Autodesk Inventor part; units mm, degrees
ref_plane "YZ Plane" through (0, 0, 0) normal (1, 0, 0) x (0, 1, 0)
ref_plane "XZ Plane" through (0, 0, 0) normal (0, 1, 0) x (-1, 0, 0)
ref_plane "XY Plane" through (0, 0, 0) normal (0, 0, 1) x (1, 0, 0)
sketch "Sketch1" plane through (0, 0, 0) normal (1, 0, 0) x (0, 1, 0)
  line L0 (0, 0) -> (-20, 0)
  line L1 (-20, 0) -> (-20, -20)
  line L2 (-20, -20) -> (0, -20)
  line L3 (0, -20) -> (0, 0)
  line L4 (0, -20) -> (4, -20)
  line L5 (4, -20) -> (4, 0)
  line L6 (4, 0) -> (0, 0)
  line L7 (0, 0) -> (0, -20)
  line L8 (4, 0) -> (0, 0)
  line L9 (0, 0) -> (0, 4)
  line L10 (0, 4) -> (4, 4)
  line L11 (4, 4) -> (4, 0)
  line L12 (0, 4) -> (-20, 4)
  line L13 (-20, 4) -> (-20, 0)
  line L14 (-20, 0) -> (0, 0)
  line L15 (0, 0) -> (0, 4)
  dimension "d0" = 20
  dimension "d1" = 20
  dimension "d2" = 4
  dimension "d3" = 4
extrude "Extrusion1" add sketch "Sketch1" along normal blind 40 contours L6 L5 L4 L3 | L9 L10 L11 L6 | L0 L13 L12 L9
sketch "Sketch2" plane through (0, -20, 4) normal (0, 0, 1) x (1, 0, 0)
  line L0 (0, 0) -> (40, 0)
  line L1 (20, 0) -> (20, 10)
  circle A0 centre (20, 10) radius 3.25
  point P0 (0, 20)
  dimension "d6" = 10
  dimension "d7" = 6.5
extrude "Extrusion2" cut sketch "Sketch2" against normal through all
sketch "Sketch3" plane through (0, -20, 4) normal (0, 0, 1) x (1, 0, 0)
  line L0 (0, 0) -> (40, 0)
  line L1 (0, 0) -> (6, 0)
  line L2 (6, 0) -> (6, 10)
  line L3 (0, 20) -> (40, 20)
  line L4 (20, 0) -> (20, 3.9788)
  line L5 (40, 0) -> (0, 0)
  line L6 (34, 0) -> (34, 10)
  circle A0 centre (34, 10) radius 2.5
  circle A1 centre (6, 10) radius 2.5
  dimension "d10" = 6
  dimension "d11" = 10
  dimension "d12" = 5
  dimension "d13" = 5
extrude "Extrusion3" cut sketch "Sketch3" against normal blind 10
sketch "Sketch4" plane through (0, 4, 4) normal (0, 1, 0) x (1, 0, 0)
  line L0 (0, 24) -> (40, 24)
  line L1 (0, 24) -> (6, 24)
  line L2 (6, 24) -> (6, 14)
  line L3 (40, 24) -> (34, 24)
  line L4 (34, 24) -> (34, 14)
  circle A0 centre (34, 14) radius 2.5
  circle A1 centre (6, 14) radius 2.5
  point P0 (0, 4)
  dimension "d16" = 6
  dimension "d17" = 10
  dimension "d18" = 6
  dimension "d19" = 10
  dimension "d20" = 5
  dimension "d21" = 5
extrude "Extrusion4" cut sketch "Sketch4" against normal blind 10
properties part number "linac_lower_ax_mount_2"
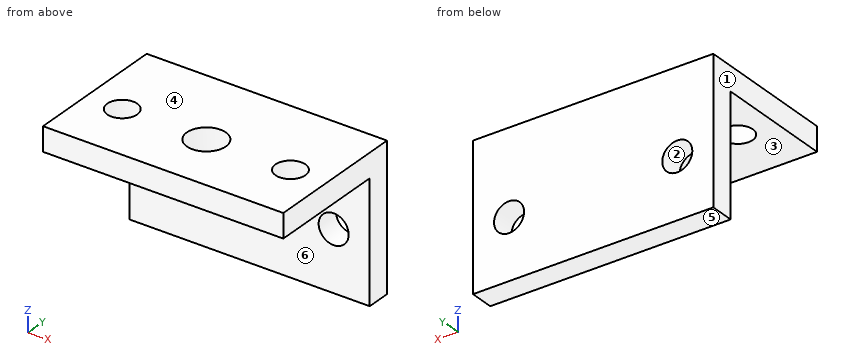
For this review, take the finished solid that the model builds, in its own axes (mm). Face numbers are marked on the shaded views. A direction names the side the tool comes from. Round coordinates to 2 decimals unless told otherwise and drop trailing zeros. Loops run counter-clockwise (first coordinate to the right, second up) from the corner with the lowest first, then second, coordinate; pieces in that order, holes last. Notation, with made-up numbers: (87, -28.5) - (106, -28.5) arc R8 cw to (106, -18.5) - close; hole circle Ø2 at (78, 53). An arc over 180 degrees is marked (long way). Use one line per item in the form item = value.
1) Tool access review of the marked faces 5 and 6: name each direction out of +Z, -Z, +X, -X, +Y, -Y from which nothing blocks a thin tool from reaching the whole face with its end or side.
Solutions:
face_5 = -Z, +X, -X, +Y, -Y
face_6 = -Z, +X, -X, -Y
2) We need section D-D on x = 34. Write out the cut boundary in (y, z).
Solutions:
outline = (-20, 0) - (-12.5, 0) - (-12.5, 4) - (-20, 4) - close; (-7.5, 0) - (0, 0) - (0, -7.5) - (4, -7.5) - (4, 4) - (-7.5, 4) - close; (0, -20) - (4, -20) - (4, -12.5) - (0, -12.5) - close
3) Mouldability with a two-part tool opening along Z and no side actions: class the marked faces 1, 2, 3 and 4 as pulls with the +Z half, pulls with the -Z half, needs draft (parallel to the pull), parting line crosses it, or undercut.
Solutions:
face_1 = needs draft
face_2 = undercut
face_3 = pulls with the -Z half
face_4 = pulls with the +Z half
4) We need section C-C on z = -10. Write out the cut boundary in (x, y).
Solutions:
outline = (0, 0) - (3.5, 0) - (3.5, 4) - (0, 4) - close; (8.5, 0) - (31.5, 0) - (31.5, 4) - (8.5, 4) - close; (36.5, 0) - (40, 0) - (40, 4) - (36.5, 4) - close
5) We need section A-A on y = -10. Write out the cut boundary in (x, z).
Solutions:
outline = (0, 0) - (3.5, 0) - (3.5, 4) - (0, 4) - close; (8.5, 0) - (16.75, 0) - (16.75, 4) - (8.5, 4) - close; (23.25, 0) - (31.5, 0) - (31.5, 4) - (23.25, 4) - close; (36.5, 0) - (40, 0) - (40, 4) - (36.5, 4) - close
6) Clearance check with flat-ended pins moving along their axes: P1, Ø10, axis at x = 24, y = -14.5, coming from the -Z side; P2, Ø5, axis at x = 13.5, z = -16, coming from the -Y side; P3, Ø3, axis at x = 34, y = -10, coming from the +Z side. State where each tip first meets the part, or that it passes through.
Solutions:
P1 = 0
P2 = 0
P3 = through
7) We need section B-B on x = 20. Write out the cut boundary in (y, z).
Solutions:
outline = (-20, 0) - (-13.25, 0) - (-13.25, 4) - (-20, 4) - close; (-6.75, 0) - (0, 0) - (0, -20) - (4, -20) - (4, 4) - (-6.75, 4) - close
8) Wall thickness on probe 1 along X at (y, z) = (1.55, -10); probe 2 along X at (y, z) = (-10, 2.45); probe 3 along Y at (x, z) = (6, 3.2): over which ranges is each line inside the solid? List them lowest first.
Solutions:
probe_1 = 0 to 3.5, 8.5 to 31.5, 36.5 to 40
probe_2 = 0 to 3.5, 8.5 to 16.75, 23.25 to 31.5, 36.5 to 40
probe_3 = -20 to -12.5, -7.5 to 4
